Geometry: final body of the model. Coordinates: model frame, mm. Face numbers are marked on the shaded views. A direction names the side the tool comes from. Round coordinates to 2 decimals unless told otherwise and drop trailing zeros. Write each loop counter-clockwise with the first axis right and the second up, starting at its lowest first coordinate (ties: lowest second). Pieces come first, ordered by that corner, then holes. Notation, with made-up numbers: (28.5, 67.25) -> (38.5, 67.25) arc R18 cw to (38.5, 99.25) -> close; hole circle Ø6 at (38, -12.75). An arc over 180 degrees is marked (long way). Use one line per item in the form item = value. Start each with the question number.
1. Cut plane A-A, the plane z = 100. Return the cut outline in (x, y), plus the area to 3 significant figures.
2. Cut plane B-B, the plane z = 263. Return the cut outline in (x, y), plus the area to 3 significant figures.
3. Reachability of the marked faces 5, 6, 7, 8 and 9 from +Z, -Z, +X, -X, +Y, -Y: full face, straight path, thin tool, end or side. Return the list, or none.
4. Draft query along Z for the marked faces 1, 2, 3 and 4. Return one class per face: pulls with the +Z half, pulls with the -Z half, needs draft (parallel to the pull), parting line crosses it, or undercut.
5. Line query: L1, parallel to X at y = -73, z = 200; L2, parallel to X at y = -75.25, z = 200; L3, parallel to Z at x = -2, y = -79. Output: solid intervals per line, ascending.
6. Pin query (flat end, axial travel): pin 1 Ø5 at (x, z) = (0, 13) entering from +Y; pin 2 Ø15.5 at (x, y) = (76.22, 31.57) entering from -Z; pin 3 Ø2 at (y, z) = (37.5, 100.5) entering from +X. Return the tip coordinate at first contact, or that it passes through.
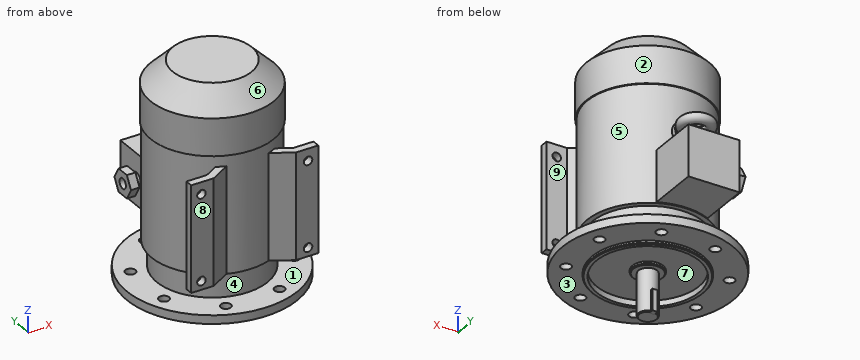
```python
from build123d import *

# Parameters (mm, degrees)
SKETCH_1_R           = 11
EXTRUDE_1_DEPTH      = 50
SKETCH_2_W           = 6
SKETCH_2_H           = 6
EXTRUDE_2_DEPTH      = 0.1
EXTRUDE_2_DEPTH_BACK = 25
CHAMFER_1_SIZE       = 1
SKETCH_3_R           = 100
EXTRUDE_3_DEPTH      = 10
SKETCH_4_R           = 65
SKETCH_4_R_2         = 60
EXTRUDE_4_DEPTH      = 3.5
SKETCH_5_R           = 60
SKETCH_5_R_2         = 18
CUT_EXTRUDE_1_DEPTH  = 3.5
CHAMFER_2_SIZE       = 1
SKETCH_6_R           = 65
EXTRUDE_5_DEPTH      = 30
SKETCH_7_R           = 71
EXTRUDE_6_DEPTH      = 137
SKETCH_8_R           = 72.248091185
EXTRUDE_7_DEPTH      = 69.5
CHAMFER_3_SIZE       = 26
SKETCH_9_R           = 6
CUT_EXTRUDE_2_DEPTH  = 247.5
EXTRUDE_8_DEPTH      = 124
CUT_EXTRUDE_3_REACH  = 182
SKETCH_11_R          = 5
SKETCH_12_W          = 60
SKETCH_12_H          = 60
EXTRUDE_9_DEPTH      = 124.5
SKETCH_13_R          = 15
EXTRUDE_10_DEPTH     = 76.5
CHAMFER_4_SIZE       = 1
SKETCH_15_R          = 6
SKETCH_16_R          = 8
EXTRUDE_11_DEPTH     = 6
EXTRUDE_12_DEPTH     = 10
SKETCH_18_R          = 6
CUT_EXTRUDE_4_DEPTH  = 10


with BuildPart() as part:
    # Эскиз1 → Вытянуть1 (new body)
    with BuildSketch(Plane.XY):
        Circle(SKETCH_1_R)
    extrude(amount=EXTRUDE_1_DEPTH)

    # Эскиз2 → Вытянуть2 (add, two sides)
    with BuildSketch(Plane(origin=(0, 0, 0), x_dir=(-1, 0, 0), z_dir=(0, 0, -1))) as extrude_2_sk:
        with Locations((0, 10.5)):
            Rectangle(SKETCH_2_W, SKETCH_2_H)
    extrude(amount=EXTRUDE_2_DEPTH)
    extrude(extrude_2_sk.sketch, amount=-EXTRUDE_2_DEPTH_BACK)

    # Фаска1
    chamfer_1_edges = [part.edges().sort_by_distance(p)[0] for p in [
        (-6.633249581, -8.774964387, 0),
    ]]
    chamfer(chamfer_1_edges, length=CHAMFER_1_SIZE)

    # Эскиз3 → Вытянуть3 (add)
    with BuildSketch(Plane.XY.offset(50)):
        Circle(SKETCH_3_R)
    extrude(amount=EXTRUDE_3_DEPTH)

    # Эскиз4 → Вытянуть4 (add)
    with BuildSketch(Plane(origin=(0, 0, 50), x_dir=(-1, 0, 0), z_dir=(0, 0, -1))):
        with Locations(Location((0, 0, 0), (0, 0, 180))):  # turned: the seam where the file's is
            Circle(SKETCH_4_R)
        Circle(SKETCH_4_R_2, mode=Mode.SUBTRACT)
    extrude(amount=EXTRUDE_4_DEPTH)

    # Эскиз5 → Вырез-Вытянуть1 (cut)
    with BuildSketch(Plane(origin=(0, 0, 50), x_dir=(-1, 0, 0), z_dir=(0, 0, -1))):
        Circle(SKETCH_5_R)
        Circle(SKETCH_5_R_2, mode=Mode.SUBTRACT)
    extrude(amount=-CUT_EXTRUDE_1_DEPTH, mode=Mode.SUBTRACT)

    # Фаска2
    chamfer_2_edges = [part.edges().sort_by_distance(p)[0] for p in [
        (-65, 0, 46.5),
        (18, 0, 50),
    ]]
    chamfer(chamfer_2_edges, length=CHAMFER_2_SIZE)

    # Эскиз6 → Вытянуть5 (add)
    with BuildSketch(Plane.XY.offset(60)):
        Circle(SKETCH_6_R)
    extrude(amount=EXTRUDE_5_DEPTH)

    # Эскиз7 → Вытянуть6 (add)
    with BuildSketch(Plane.XY.offset(90)):
        Circle(SKETCH_7_R)
    extrude(amount=EXTRUDE_6_DEPTH)

    # Эскиз8 → Вытянуть7 (add)
    with BuildSketch(Plane.XY.offset(227)):
        Circle(SKETCH_8_R)
    extrude(amount=EXTRUDE_7_DEPTH)

    # Фаска3
    chamfer_3_edges = [part.edges().sort_by_distance(p)[0] for p in [
        (-72.248091185, 0, 296.5),
    ]]
    chamfer(chamfer_3_edges, length=CHAMFER_3_SIZE)

    # Эскиз9 → Вырез-Вытянуть2 (cut, through all)
    with BuildSketch(Plane(origin=(0, 0, 50), x_dir=(-1, 0, 0), z_dir=(0, 0, -1))):
        with Locations((-31.57138317, 76.220061432)):
            Circle(SKETCH_9_R)
        with Locations((31.57138317, 76.220061432)):
            Circle(SKETCH_9_R)
        with Locations((76.220061432, 31.57138317)):
            Circle(SKETCH_9_R)
        with Locations((76.220061432, -31.57138317)):
            Circle(SKETCH_9_R)
        with Locations((31.57138317, -76.220061432)):
            Circle(SKETCH_9_R)
        with Locations((-31.57138317, -76.220061432)):
            Circle(SKETCH_9_R)
        with Locations((-76.220061432, -31.57138317)):
            Circle(SKETCH_9_R)
        with Locations((-76.220061432, 31.57138317)):
            Circle(SKETCH_9_R)
    extrude(amount=-CUT_EXTRUDE_2_DEPTH, mode=Mode.SUBTRACT)

    # Эскиз10 → Вытянуть8 (add)
    with BuildSketch(Plane(origin=(0, 0, 90), x_dir=(-1, 0, 0), z_dir=(0, 0, -1))):
        Polygon((-74.5, -80), (-48.088457268, -80), (-11.515477308, -58.884580175), (-23.295059446, -55.293220248), (-50.5, -71), (-74.5, -71), align=None)
        Polygon((74.5, -71), (74.5, -80), (48.088457268, -80), (11.515477308, -58.884580175), (23.295059446, -55.293220248), (50.5, -71), align=None)
    extrude(amount=-EXTRUDE_8_DEPTH)

    # Эскиз11 → Вырез-Вытянуть3 (cut, up to next)
    with BuildSketch(Plane.XZ.offset(80), mode=Mode.PRIVATE) as cut_extrude_3_sk1:
        with Locations(Location((-62.5, 100, 0), (0, 0, 270))):  # turned: the seam where the file's is
            Circle(SKETCH_11_R)
    cut_extrude_3_tool1 = extrude(cut_extrude_3_sk1.sketch, amount=-CUT_EXTRUDE_3_REACH, mode=Mode.PRIVATE) & part.part
    add(cut_extrude_3_tool1.solids().sort_by_distance((-62.5, -80, 100))[0], mode=Mode.SUBTRACT)
    # Эскиз11 → Вырез-Вытянуть3 (cut, up to next)
    with BuildSketch(Plane.XZ.offset(80), mode=Mode.PRIVATE) as cut_extrude_3_sk2:
        with Locations(Location((62.5, 100, 0), (0, 0, 270))):  # turned: the seam where the file's is
            Circle(SKETCH_11_R)
    cut_extrude_3_tool2 = extrude(cut_extrude_3_sk2.sketch, amount=-CUT_EXTRUDE_3_REACH, mode=Mode.PRIVATE) & part.part
    add(cut_extrude_3_tool2.solids().sort_by_distance((62.5, -80, 100))[0], mode=Mode.SUBTRACT)
    # Эскиз11 → Вырез-Вытянуть3 (cut, up to next)
    with BuildSketch(Plane.XZ.offset(80), mode=Mode.PRIVATE) as cut_extrude_3_sk3:
        with Locations(Location((-62.5, 200, 0), (0, 0, 270))):  # turned: the seam where the file's is
            Circle(SKETCH_11_R)
    cut_extrude_3_tool3 = extrude(cut_extrude_3_sk3.sketch, amount=-CUT_EXTRUDE_3_REACH, mode=Mode.PRIVATE) & part.part
    add(cut_extrude_3_tool3.solids().sort_by_distance((-62.5, -80, 200))[0], mode=Mode.SUBTRACT)
    # Эскиз11 → Вырез-Вытянуть3 (cut, up to next)
    with BuildSketch(Plane.XZ.offset(80), mode=Mode.PRIVATE) as cut_extrude_3_sk4:
        with Locations(Location((62.5, 200, 0), (0, 0, 270))):  # turned: the seam where the file's is
            Circle(SKETCH_11_R)
    cut_extrude_3_tool4 = extrude(cut_extrude_3_sk4.sketch, amount=-CUT_EXTRUDE_3_REACH, mode=Mode.PRIVATE) & part.part
    add(cut_extrude_3_tool4.solids().sort_by_distance((62.5, -80, 200))[0], mode=Mode.SUBTRACT)

    # Эскиз12 → Вытянуть9 (add)
    with BuildSketch(Plane(origin=(0, 0, 0), x_dir=(1, 0, 0), z_dir=(0, 1, 0))):
        with Locations((0, -121)):
            Rectangle(SKETCH_12_W, SKETCH_12_H)
    extrude(amount=EXTRUDE_9_DEPTH)

    # Эскиз13 → Вытянуть10 (add)
    with BuildSketch(Plane(origin=(0, 0, 0), x_dir=(1, 0, 0), z_dir=(0, 1, 0))):
        with Locations(Location((0, -175, 0), (0, 0, 90))):  # turned: the seam where the file's is
            Circle(SKETCH_13_R)
    extrude(amount=EXTRUDE_10_DEPTH)

    # Фаска4
    chamfer_4_edges = [part.edges().sort_by_distance(p)[0] for p in [
        (0, 76.5, 190),
    ]]
    chamfer(chamfer_4_edges, length=CHAMFER_4_SIZE)

    # По траектории1: sweep along a path in Эскиз14
    with BuildLine(Plane.XY.offset(175)) as sweep_1_path:
        CenterArc((0, 91.5), 15, 0, 360)
    # Эскиз15 → По траектории1 (sweep)
    with BuildSketch(Plane(origin=(0, 0, 0), x_dir=(0, 0, -1), z_dir=(1, 0, 0))):
        with Locations((-175, 106.5)):
            Circle(SKETCH_15_R)
    sweep(path=sweep_1_path.line)

    # Эскиз16 → Вытянуть11 (add)
    with BuildSketch(Plane.ZY.offset(30)):
        with Locations(Location((121, 94.5, 0), (0, 0, 180))):  # turned: the seam where the file's is
            Circle(SKETCH_16_R)
    extrude(amount=EXTRUDE_11_DEPTH)

    # Эскиз17 → Вытянуть12 (add)
    with BuildSketch(Plane.ZY.offset(36)):
        Polygon((121, 110.088457268), (107.5, 102.294228634), (107.5, 86.705771366), (121, 78.911542732), (134.5, 86.705771366), (134.5, 102.294228634), align=None)
    extrude(amount=EXTRUDE_12_DEPTH)

    # Эскиз18 → Вырез-Вытянуть4 (cut)
    with BuildSketch(Plane.ZY.offset(46)):
        with Locations((121, 94.5)):
            Circle(SKETCH_18_R)
    extrude(amount=-CUT_EXTRUDE_4_DEPTH, mode=Mode.SUBTRACT)


solid = part.part
```
Outcome:
q1.outline = (-74.5, -80) -> (-67.5, -80) -> (-67.5, -71) -> (-74.5, -71) -> close; (-57.5, -80) -> (-48.09, -80) -> (-24.77, -66.54) arc R71 ccw to (24.77, -66.54) -> (48.09, -80) -> (57.5, -80) -> (57.5, -71) -> (50.5, -71) -> (34.76, -61.91) arc R71 ccw to (30, 64.35) -> (30, 124.5) -> (-30, 124.5) -> (-30, 64.35) arc R71 ccw to (-34.76, -61.91) -> (-50.5, -71) -> (-57.5, -71) -> close; (67.5, -80) -> (74.5, -80) -> (74.5, -71) -> (67.5, -71) -> close
q1.area = 19,900 mm^2
q2.outline = circle Ø144.5 at (0, 0)
q2.area = 16,400 mm^2
q3.face_5 = none
q3.face_6 = +Z
q3.face_7 = -Z
q3.face_8 = +Z, +X, -X, -Y
q3.face_9 = +Z, +X
q4.face_1 = undercut
q4.face_2 = needs draft
q4.face_3 = pulls with the -Z half
q4.face_4 = undercut
q5.L1 = -74.5 to -67.5, -57.5 to -35.96, 35.96 to 57.5, 67.5 to 74.5
q5.L2 = -74.5 to -67.5, -57.5 to -39.86, 39.86 to 57.5, 67.5 to 74.5
q5.L3 = 50 to 60
q6.pin_1 = 13.5
q6.pin_2 = 50
q6.pin_3 = 60.9
